Source: CAD feature listing. Evaluate the final solid. Frame: model axes, mm. A direction names the side the tool comes from. Coordinates: 2 decimals unless noted, no trailing zeros. Loops run counter-clockwise (first coordinate to the right, second up) from the corner with the lowest first, then second, coordinate; pieces in that order, holes last.
Item 1: Reachability of faces 5 (the flat face through (0, 0, 2.7)), 6 (the flat face through (0, 0, 0.2)), 7 (the flat face through (4.7, 2.5, 0.25)) from +Z, -Z, +X, -X, +Y, -Y: full face, straight path, thin tool, end or side. Return the list, or none.
Item 2: Line query: probe 1 along X at (y, z) = (-2.75, 1.3); probe 2 along X at (y, z) = (-2.5, 1.1); probe 3 along Z at (x, y) = (1, 1.75). Output: solid intervals per line, ascending.
Item 3: Pull-direction query (Y, two-part tool) for faces 1 (the flat face through (0, 4.15, 1)), 2 (the flat face through (-3.89, -1.89, 0.69)), 3 (the flat face through (0, -4.15, 1)), 4 (the flat face through (-4.5, 2.5, 0)); classes: +Y half, -Y half, draft (parallel to the pull), parting line (faces both ways), or undercut.
Item 4: Pin query (flat end, axial travel): pin 1 Ø1.3 at (x, z) = (4.5, 1) entering from +Y; pin 2 Ø1.5 at (x, y) = (1.5, 0) entering from -Z; pin 3 Ø0.5 at (x, z) = (-4, 1) entering from -Y. Return the tip coordinate at first contact, or that it passes through.
Item 5: Section query C-C, the plane x = 2.75. Return the cut outline in (y, z), then the cut area to 3 significant figures.
Item 6: Section query A-A, the plane z = 0.9. Return the cut outline in (x, y).
Item 7: Section query D-D, the plane y = 0.75. Return the cut outline in (x, z).
Item 8: Section query B-B, the plane y = 2.25. Return the cut outline in (x, z).
```python
from build123d import *

# Parameters (mm, degrees)
PAD002_DEPTH = 0.65
PAD003_DEPTH = 0.65
PAD_DEPTH    = 4.15
CHAMFER_SIZE = 0.5


with BuildPart() as pad002:
    # Sketch002 → Pad002 (new body, symmetric)
    with BuildSketch(Plane.XZ.offset(-2.54)):
        Polygon((-5.1, 0), (-3.95, 0), (-3.5, 1.35), (3.5, 1.35), (3.95, 0), (5.1, 0), (5.1, 0.25), (4.2, 0.25), (3.75, 1.6), (-3.75, 1.6), (-4.2, 0.25), (-5.1, 0.25), align=None)
    extrude(amount=PAD002_DEPTH, both=True)


with BuildPart() as pad003:
    # Sketch003 → Pad003 (new body, symmetric)
    with BuildSketch(Plane.XZ.offset(2.54)):
        Polygon((-5.1, 0), (-3.95, 0), (-3.5, 1.35), (3.5, 1.35), (3.95, 0), (5.1, 0), (5.1, 0.25), (4.2, 0.25), (3.75, 1.6), (-3.75, 1.6), (-4.2, 0.25), (-5.1, 0.25), align=None)
    extrude(amount=PAD003_DEPTH, both=True)


with BuildPart() as obj1:
    # Sketch → Pad (new body, symmetric)
    with BuildSketch(Plane.XZ):
        Polygon((-3.1, 0.2), (3.1, 0.2), (3.25, 1.45), (3.1, 2.7), (-3.1, 2.7), (-3.25, 1.45), align=None)
    extrude(amount=PAD_DEPTH, both=True)

    # Chamfer
    chamfer_edges = [obj1.edges().sort_by_distance(p)[0] for p in [
        (0, 4.15, 2.7),
    ]]
    chamfer(chamfer_edges, length=CHAMFER_SIZE)

    add(pad002.part)
    add(pad003.part)


solid = obj1.part
```
Verdict:
1. face 5: +Z, +X, -X, +Y, -Y
1. face 6: -Z, +Y, -Y
1. face 7: +Z, +X, +Y, -Y
2. probe 1: x = -3.85 to -3.52, -3.23 to 3.23, 3.52 to 3.85
2. probe 2: x = -3.92 to -3.58, -3.21 to 3.21, 3.58 to 3.92
2. probe 3: z = 0.2 to 2.7
3. face 1: +Y half
3. face 2: undercut
3. face 3: -Y half
3. face 4: draft
4. pin 1: stops at y = 3.19
4. pin 2: stops at z = 0.2
4. pin 3: stops at y = -3.19
5. outline: (-4.15, 0.2) - (4.15, 0.2) - (4.15, 2.2) - (3.65, 2.7) - (-4.15, 2.7) - close
5. area: 20.6 mm2
6. outline: (-3.98, -3.19) - (-3.65, -3.19) - (-3.65, -1.89) - (-3.98, -1.89) - close; (-3.98, 1.89) - (-3.65, 1.89) - (-3.65, 3.19) - (-3.98, 3.19) - close; (-3.18, -4.15) - (3.18, -4.15) - (3.18, 4.15) - (-3.18, 4.15) - close; (3.65, -3.19) - (3.98, -3.19) - (3.98, -1.89) - (3.65, -1.89) - close; (3.65, 1.89) - (3.98, 1.89) - (3.98, 3.19) - (3.65, 3.19) - close
7. outline: (-3.25, 1.45) - (-3.1, 0.2) - (3.1, 0.2) - (3.25, 1.45) - (3.1, 2.7) - (-3.1, 2.7) - close
8. outline: (-5.1, 0) - (-3.95, 0) - (-3.5, 1.35) - (-3.24, 1.35) - (-3.1, 0.2) - (3.1, 0.2) - (3.24, 1.35) - (3.5, 1.35) - (3.95, 0) - (5.1, 0) - (5.1, 0.25) - (4.2, 0.25) - (3.75, 1.6) - (3.23, 1.6) - (3.1, 2.7) - (-3.1, 2.7) - (-3.23, 1.6) - (-3.75, 1.6) - (-4.2, 0.25) - (-5.1, 0.25) - close
